from build123d import *
from OCP.BRepFilletAPI import BRepFilletAPI_MakeChamfer

# Parameters (mm, degrees)
SKETCH_1_W          = 29.6
SKETCH_1_H          = 9
EXTRUDE_1_DEPTH     = 4.5
CUT_EXTRUDE_1_DEPTH = 3
SKETCH_3_W          = 1.5
SKETCH_3_H          = 4
EXTRUDE_2_DEPTH     = 7
SKETCH_4_W          = 2
SKETCH_4_H          = 2
CUT_EXTRUDE_2_DEPTH = 23.230384612
CHAMFER_1_SIZE      = 1
CHAMFER_1_SIZE2     = 1.732050808
CHAMFER_2_SIZE      = 1
CHAMFER_2_SIZE2     = 1.732050808
CUT_EXTRUDE_3_DEPTH = 31.276393444
FILLET_2_R          = 0.2
FILLET_3_R          = 0.5


with BuildPart() as part:
    # 草图1 → 凸台-拉伸1 (new body)
    with BuildSketch(Plane(origin=(0, 0, 0), x_dir=(1, 0, 0), z_dir=(0, 1, 0))):
        Rectangle(SKETCH_1_W, SKETCH_1_H)
    extrude(amount=EXTRUDE_1_DEPTH)

    # 草图2 → 切除-拉伸1 (cut)
    with BuildSketch(Plane.XZ):
        Polygon((-13.3, 0.5), (-13.3, 3), (13.3, 3), (13.3, 0.5), (6.5, 0.5), (6.5, -0.5), (13.3, -0.5), (13.3, -3), (-13.3, -3), (-13.3, -0.5), (-6.5, -0.5), (-6.5, 0.5), align=None)
    extrude(amount=-CUT_EXTRUDE_1_DEPTH, mode=Mode.SUBTRACT)

    # 草图3 → 凸台-拉伸2 (add)
    with BuildSketch(Plane.XZ.offset(-3)):
        with Locations((-5.75, 0)):
            Rectangle(SKETCH_3_W, SKETCH_3_H)
        with Locations((5.75, 0)):
            Rectangle(SKETCH_3_W, SKETCH_3_H)
    extrude(amount=EXTRUDE_2_DEPTH)

    # 草图4 → 切除-拉伸2 (cut, through all)
    with BuildSketch(Plane.ZY.offset(6.5)):
        with Locations((0, -2)):
            Rectangle(SKETCH_4_W, SKETCH_4_H)
    extrude(amount=-CUT_EXTRUDE_2_DEPTH, mode=Mode.SUBTRACT)

    # 倒角1: one chamfer whose edges measure the first distance from different faces: ONE call of the kernel's chamfer builder (chamfer() names one face for all edges)
    chamfer_1_edges_1 = [part.edges().sort_by_distance(p)[0] for p in [
        (0, 4.5, -4.5),
    ]]
    chamfer_1_side_1 = [part.faces().sort_by_distance(p)[0] for p in [
        (0, 2.25, -4.5),
    ]]
    chamfer_1_edges_2 = [part.edges().sort_by_distance(p)[0] for p in [
        (0, 4.5, 4.5),
    ]]
    chamfer_1_side_2 = [part.faces().sort_by_distance(p)[0] for p in [
        (0, 2.25, 4.5),
    ]]
    chamfer_1 = BRepFilletAPI_MakeChamfer(part.part.solid().wrapped)
    for e in chamfer_1_edges_1:
        chamfer_1.Add(CHAMFER_1_SIZE, CHAMFER_1_SIZE2, e.wrapped, chamfer_1_side_1[0].wrapped)  # the first distance lies on this face
    for e in chamfer_1_edges_2:
        chamfer_1.Add(CHAMFER_1_SIZE, CHAMFER_1_SIZE2, e.wrapped, chamfer_1_side_2[0].wrapped)  # the first distance lies on this face
    add(Compound.cast(chamfer_1.Shape()), mode=Mode.REPLACE)

    # 倒角2: one chamfer whose edges measure the first distance from different faces: ONE call of the kernel's chamfer builder (chamfer() names one face for all edges)
    chamfer_2_edges_1 = [part.edges().sort_by_distance(p)[0] for p in [
        (-14.8, 4.5, 0),
    ]]
    chamfer_2_side_1 = [part.faces().sort_by_distance(p)[0] for p in [
        (-14.8, 2.164368335, 0),
    ]]
    chamfer_2_edges_2 = [part.edges().sort_by_distance(p)[0] for p in [
        (14.8, 4.5, 0),
    ]]
    chamfer_2_side_2 = [part.faces().sort_by_distance(p)[0] for p in [
        (14.8, 2.164368335, 0),
    ]]
    chamfer_2 = BRepFilletAPI_MakeChamfer(part.part.solid().wrapped)
    for e in chamfer_2_edges_1:
        chamfer_2.Add(CHAMFER_2_SIZE, CHAMFER_2_SIZE2, e.wrapped, chamfer_2_side_1[0].wrapped)  # the first distance lies on this face
    for e in chamfer_2_edges_2:
        chamfer_2.Add(CHAMFER_2_SIZE, CHAMFER_2_SIZE2, e.wrapped, chamfer_2_side_2[0].wrapped)  # the first distance lies on this face
    add(Compound.cast(chamfer_2.Shape()), mode=Mode.REPLACE)

    # 草图5 → 切除-拉伸3 (cut, through all)
    with BuildSketch(Plane.ZY.offset(14.8)):
        Polygon((-1.25, 4.5), (-0.25, 4.5), (-0.75, 4.2), align=None)
        Polygon((0.75, 4.2), (1.25, 4.5), (0.25, 4.5), align=None)
    extrude(amount=-CUT_EXTRUDE_3_DEPTH, mode=Mode.SUBTRACT)

    # 圆角2
    fillet_2_edges = [part.edges().sort_by_distance(p)[0] for p in [
        (-14.8, 1.75, 4.5),
        (-14.8, 1.75, -4.5),
        (14.8, 1.75, -4.5),
        (14.8, 1.75, 4.5),
        (0, 0, -4.5),
        (14.8, 0, 0),
        (0, 0, 4.5),
        (-14.8, 0, 0),
    ]]
    fillet(fillet_2_edges, radius=FILLET_2_R)

    # 圆角3
    fillet_3_edges = [part.edges().sort_by_distance(p)[0] for p in [
        (-5.75, -4, -2),
        (-5.75, -4, 2),
        (5.75, -4, -2),
        (5.75, -4, 2),
    ]]
    fillet(fillet_3_edges, radius=FILLET_3_R)


solid = part.part
Work out the finished part from the listing and answer in its coordinate system (mm). A direction names the side the tool comes from. Coordinates: 2 decimals unless noted, no trailing zeros. Write each loop counter-clockwise with the first axis right and the second up, starting at its lowest first coordinate (ties: lowest second). Pieces come first, ordered by that corner, then holes. Notation, with made-up numbers: M -22,-29.75 L -7,-29.75 A25 cw -7,-16.75 Z; hole C 17.25,3 d2. An arc over 180 degrees is marked long. Answer as CSV lines item,"result". Start each with the question number.
Item 1: Section A-A on y = -2.25 is taken. Write down the section's boundary in (x, z).
Item 2: Section D-D on x = 3.5 is taken. Write down the section's boundary in (y, z), and give its area (3 significant figures).
Item 3: Section C-C on y = -0.5 is taken. Write down the section's boundary in (x, z).
Item 4: A tool of negligible diameter and unlimited length cuts with its end or side. For faces 1 (the face through (0, 2, 4.5)), 2 (the face through (-10, 1, 0.5)), 3 (the face through (-6, -3, 0)), from which of +Z, -Z, +X, -X, +Y, -Y can it reach the whole face along a straight path? Write none if from no direction.
Item 5: Consider L1, parallel to Z at x = 8.5, y = 1.75; L2, parallel to X at y = 0.25, z = -0.75; L3, parallel to Z at x = -2.75, y = 1.5. Determine where each line is inside the solid, lowest interval first.
Item 6: Determine the mould class of faces 4 (the face through (-0.1, 0, 3.2)), 5 (the face through (-6, -2, -1)), 6 (the face through (0, 1, -3)) for opening direction Y: released by +Y, released by -Y, zero draft, split by the parting line, or undercut.
Item 7: Flat-ended cylindrical pins translate along their axes: P1, Ø1.6, axis at x = 6, y = -2, coming from the +Z side; P2, Ø0.8, axis at x = 5.5, y = -2.5, coming from the -Z side; P3, Ø2, axis at y = -0.5, z = -2.5, coming from the -X side; P4, Ø2, axis at x = 8, z = 3.5, coming from the -Y side. Find the tip coordinate at first contact, or state that the pin passes through.
Item 8: Section B-B on x = -6 is taken. Write down the section's boundary in (y, z), and give its area (3 significant figures).
Checks:
1,outline,"M -6.5,-2 L -5,-2 L -5,-1 L -6.5,-1 Z; M -6.5,1 L -5,1 L -5,2 L -6.5,2 Z; M 5,-2 L 6.5,-2 L 6.5,-1 L 5,-1 Z; M 5,1 L 6.5,1 L 6.5,2 L 5,2 Z"
2,outline,"M 0,-4.3 A0.2 ccw 0.2,-4.5 L 3.5,-4.5 L 4.5,-2.77 L 4.5,-1.25 L 4.2,-0.75 L 4.5,-0.25 L 4.5,0.25 L 4.2,0.75 L 4.5,1.25 L 4.5,2.77 L 3.5,4.5 L 0.2,4.5 A0.2 ccw 0,4.3 L 0,3 L 3,3 L 3,-3 L 0,-3 Z"
2,area,"20.5 mm²"
3,outline,"M -6.5,-2 L -5,-2 L -5,2 L -6.5,2 Z; M 5,-2 L 6.5,-2 L 6.5,2 L 5,2 Z"
4,face 1,"+Z, +X, -X, +Y, -Y"
4,face 2,"-Y"
4,face 3,"+X, -X"
5,L1,"z = -4.5 to -3, -0.5 to 0.5, 3 to 4.5"
5,L2,"x = -14.8 to -13.3, -6.5 to -5, 5 to 6.5, 13.3 to 14.8"
5,L3,"z = -4.5 to -3, 3 to 4.5"
6,face 4,"released by -Y"
6,face 5,"undercut"
6,face 6,"zero draft"
7,P1,"stops at z = 2"
7,P2,"stops at z = -2"
7,P3,"stops at x = -14.8"
7,P4,"stops at y = 0"
8,outline,"M -4,-1.5 A0.5 ccw -3.5,-2 L 3,-2 L 3,-3 L 0,-3 L 0,-4.3 A0.2 ccw 0.2,-4.5 L 3.5,-4.5 L 4.5,-2.77 L 4.5,-1.25 L 4.2,-0.75 L 4.5,-0.25 L 4.5,0.25 L 4.2,0.75 L 4.5,1.25 L 4.5,2.77 L 3.5,4.5 L 0.2,4.5 A0.2 ccw 0,4.3 L 0,3 L 3,3 L 3,2 L -3.5,2 A0.5 ccw -4,1.5 Z; hole M -3,-1 L -1,-1 L -1,1 L -3,1 Z"
8,area,"44.3 mm²"
